```python
from build123d import *

# Parameters (mm, degrees)
BASEEXTRUDE_DEPTH   = 2
SKETCH1_R           = 2
CUT_EXTRUDE1_DEPTH  = 3
SKETCH2_R           = 2.45
BOSS_EXTRUDE1_DEPTH = 2
FILLET1_R           = 1


with BuildPart() as part:
    # BaseSketch → BaseExtrude (new body)
    with BuildSketch(Plane(origin=(0, 0, 0), x_dir=(1, 0, 0), z_dir=(0, 1, 0))):
        with BuildLine():
            Line((35, 15), (0, 15))
            ThreePointArc((0, 15), (-8.660254038, -12.247448714), (14.142135624, 5))
            Line((14.142135624, 5), (45, 5))
            Line((45, 5), (85.857864376, 5))
            ThreePointArc((85.857864376, 5), (108.660254038, -12.247448714), (100, 15))
            Line((100, 15), (45, 15))
            Line((45, 15), (45, 60))
            ThreePointArc((45, 60), (17.752551286, 68.660254038), (35, 45.857864376))
            Line((35, 45.857864376), (35, 15))
        make_face()
    extrude(amount=BASEEXTRUDE_DEPTH)

    # Sketch1 → Cut-Extrude1 (cut, through all)
    with BuildSketch(Plane.XZ):
        with Locations((40, -10)):
            Circle(SKETCH1_R)
    extrude(amount=-CUT_EXTRUDE1_DEPTH, mode=Mode.SUBTRACT)

    # Sketch2 → Boss-Extrude1 (add)
    with BuildSketch(Plane.XZ):
        with Locations((40, -16.5)):
            Circle(SKETCH2_R)
    extrude(amount=BOSS_EXTRUDE1_DEPTH)

    # Fillet1
    fillet1_edges = [part.edges().sort_by_distance(p)[0] for p in [
        (37.55, -2, -16.5),
    ]]
    fillet(fillet1_edges, radius=FILLET1_R)


solid = part.part
```
For this review, take the finished solid that the model builds, in its own axes (mm). Round coordinates to 2 decimals unless told otherwise and drop trailing zeros. Order: outer loops, then holes, each group sorted by start corner. A loop starts at its lowest first (then second) coordinate and runs counter-clockwise, first axis right, second up. Notation, with made-up numbers: (44.25, 8.25) -> (78.25, 8.25) arc R11 ccw to (78.25, 27.25) -> close; hole circle Ø11 at (1.5, -26.5). An arc over 180 degrees is marked (long way). Use a Markdown table: item, result.
Item 1: Take a section at C-C (x = 30). State the section outline as (y, z) points.
Resolved:
| item | result |
|---|---|
| outline | (0, -75) -> (2, -75) -> (2, -45) -> (0, -45) -> close; (0, -15) -> (2, -15) -> (2, -5) -> (0, -5) -> close |
Item 2: Take a section at B-B (z = 0). State the section outline as (x, y) points, plus the area to 3 significant figures.
Resolved:
| item | result |
|---|---|
| outline | (-15, 0) -> (15, 0) -> (15, 2) -> (-15, 2) -> close; (85, 0) -> (115, 0) -> (115, 2) -> (85, 2) -> close |
| area | 120 mm² |
Item 3: For pin 1 (1.6 mm diameter, centred on x = 84.5, y = 1, fed in from -Z); pin 2 (2 mm diameter, centred on x = 62, y = 1, fed in from +Z); pin 3 (1.6 mm diameter, centred on y = 1, z = -37, fed in from -X); pin 4 (10 mm diameter, centred on x = 64, z = 1.5, fed in from -Y), all flat-tipped, find the tip position at first contact; note any pin that passes through.
Resolved:
| item | result |
|---|---|
| pin 1 | stops at z = -15 |
| pin 2 | stops at z = -5 |
| pin 3 | stops at x = 35 |
| pin 4 | passes through |
Item 4: Draft analysis for pull direction X (two halves, no side actions). For faces 1 (the cylindrical face through (108.222, 0.986, 12.546)), 2 (the cylindrical face through (42.263, -0.493, -17.438)), 3 (the flat face through (40, 2, -24)), state which applies: +X half, -X half, draft (parallel to the pull), parting line (faces both ways), or undercut.
Resolved:
| item | result |
|---|---|
| face 1 | undercut |
| face 2 | parting line |
| face 3 | draft |
Item 5: Take a section at A-A (y = 0.7). State the section outline as (x, z) points, plus the area to 3 significant figures.
Resolved:
| item | result |
|---|---|
| outline | (0, -15) -> (35, -15) -> (35, -45.86) arc R15 ccw (long way) to (45, -60) -> (45, -15) -> (100, -15) arc R15 ccw (long way) to (85.86, -5) -> (14.14, -5) arc R15 ccw (long way) to start; hole circle Ø4 at (40, -10) |
| area | 3,250 mm² |
Item 6: Take a section at D-D (x = 83). State the section outline as (y, z) points, plus the area to 3 significant figures.
Resolved:
| item | result |
|---|---|
| outline | (0, -15) -> (2, -15) -> (2, -5) -> (0, -5) -> close |
| area | 20.0 mm² |
Item 7: For line 1 along Z through (x, y) = (40, 1.1); line 2 along X through (y, z) = (0.8, -41); line 3 along Y through (x, z) = (37, -42), list the stretches that pass through material, from the lowest coordinate up. Write a range as [from, to].
Resolved:
| item | result |
|---|---|
| line 1 | z = [-71.18, -12], [-8, -5] |
| line 2 | x = [35, 45] |
| line 3 | y = [0, 2] |
